from build123d import *

# Parameters (mm, degrees)
BOSS_EXTRUDE1_DEPTH = 8
SKETCH2_R           = 2
CUT_EXTRUDE1_DEPTH  = 63.459987192
FILLET3_R           = 8
FILLET4_START       = -27.5
FILLET4_DEPTH       = 55


with BuildPart() as part:
    # Sketch1 → Boss-Extrude1 (new body)
    with BuildSketch(Plane.XY):
        Polygon((-27.5, 28.5), (-27.5, -28.5), (-10, -28.5), (-10, -20.5), (10, -20.5), (10, -28.5), (27.5, -28.5), (27.5, 28.5), align=None)
    extrude(amount=BOSS_EXTRUDE1_DEPTH)

    # Sketch2 → Cut-Extrude1 (cut, through all)
    with BuildSketch(Plane(origin=(27.5, 0, 0), x_dir=(0, 0, -1), z_dir=(1, 0, 0))):
        with Locations((-4, 21.5)):
            Circle(SKETCH2_R)
    extrude(amount=-CUT_EXTRUDE1_DEPTH, mode=Mode.SUBTRACT)

    # Fillet3
    # the kernel refuses this fillet: 8 mm, written as the material it takes off along each edge
    with BuildSketch(Plane(origin=(47.5, 28.5, 8), x_dir=(0, 0, -1), z_dir=(-1, 0, 0))) as fillet3_piece_1:
        with BuildLine():
            CenterArc((FILLET3_R, FILLET3_R), FILLET3_R, 180, 90)
            Line((0, FILLET3_R), (0, 0))
            Line((0, 0), (FILLET3_R, 0))
        make_face()
    extrude(amount=95, mode=Mode.SUBTRACT)
    with BuildSketch(Plane(origin=(47.5, 28.5, 0), x_dir=(0, 0, 1), z_dir=(-1, 0, 0))) as fillet3_piece_2:
        with BuildLine():
            CenterArc((FILLET3_R, -FILLET3_R), FILLET3_R, 90, 90)
            Line((0, -FILLET3_R), (0, 0))
            Line((0, 0), (FILLET3_R, 0))
        make_face()
    extrude(amount=95, mode=Mode.SUBTRACT)

    # Fillet4: read off the stored shape, not the designer's step
    # Fillet4 outline → Fillet4 (cut)
    with BuildSketch(Plane.YZ.offset(FILLET4_START)):
        with BuildLine():
            Line((-28.5, 8), (-28.5, 0))
            add(Edge.make_bspline(
                [(-28.5, 0), (-28.5, 8), (-16.5, 8)],
                knots=[0, 0, 0, 1, 1, 1], degree=2, weights=[1, 0.707106781, 1]))
            Line((-16.5, 8), (-28.5, 8))
        make_face()
    extrude(amount=FILLET4_DEPTH, mode=Mode.SUBTRACT)


solid = part.part
Verification items for the finished model (mm, model axes). A direction names the side the tool comes from. Coordinates: 2 decimals unless noted, no trailing zeros. Order: outer loops, then holes, each group sorted by start corner. A loop starts at its lowest first (then second) coordinate and runs counter-clockwise, first axis right, second up.
Item 1: Release check for a two-part mould opening along Y. For faces 1 (the face through (0, -20.5, 4)), 2 (the face through (0.385, 24.449, 6.957)), 3 (the face through (0.385, 22.852, 5.474)) record: +Y half, -Y half, draft (parallel to the pull), parting line (faces both ways), or undercut.
Filled in:
face 1: -Y half
face 2: +Y half
face 3: undercut
Item 2: Section check A-A, the plane y = 21.5. Enter the section's corners in (x, z).
Filled in:
outline: (-27.5, 0.06) - (27.5, 0.06) - (27.5, 2) - (-27.5, 2) - close; (-27.5, 6) - (27.5, 6) - (27.5, 7.94) - (-27.5, 7.94) - close
Item 3: Material ranges on L1, parallel to Y at x = -13.5, z = 5.75; L2, parallel to Y at x = -12, z = 5.5; L3, parallel to Z at x = -9, y = 23, recorded low to high.
Filled in:
L1: y = -24.84 to 20.53, 22.47 to 26.06
L2: y = -25.21 to 20.18, 22.82 to 26.31
L3: z = 0.4 to 2.68, 5.32 to 7.6
Item 4: Depth check by flat-ended pin: pin 1 (8 mm diameter, centred on x = 20, y = 16.5, fed in from -Z); pin 2 (1 mm diameter, centred on x = -1.5, z = 5, fed in from -Y); pin 3 (2.5 mm diameter, centred on y = 21.5, z = 4, fed in from +X); pin 4 (2 mm diameter, centred on x = -11.5, z = 5.5, fed in from +Y). Enter the tip coordinate at first touch or a pass-through.
Filled in:
pin 1: stops at z = 0
pin 2: stops at y = -20.5
pin 3: passes through
pin 4: stops at y = 27.11
Item 5: Access from +Z, -Z, +X, -X, +Y, -Y to the whole of each face (thin tool, end or side, straight path). Record for faces 4 (the face through (0.39, 24.55, 1.1)), 5 (the face through (10, -24, 3)).
Filled in:
face 4: -Z, +X, -X, +Y
face 5: +Z, -Z, -Y
